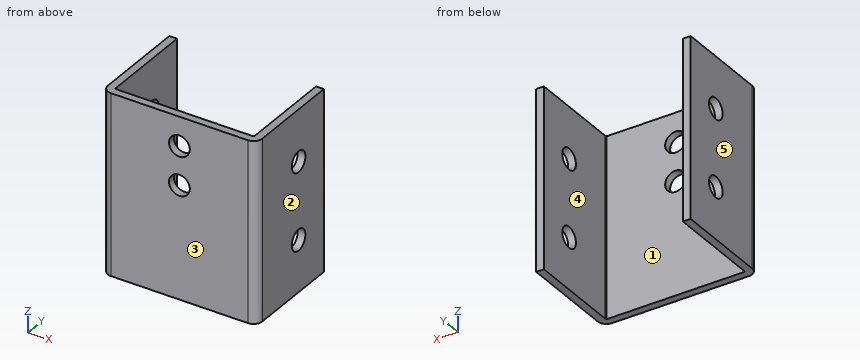
from build123d import *

# Parameters (mm, degrees)
SKETCH1_W                      = 60
SKETCH1_H                      = 70
BASE_FLANGE1_DEPTH             = 3
EDGE_FLANGE1_STRIP_W           = 12.8
EDGE_FLANGE1_STRIP_H           = 3
EDGE_FLANGE1_STRIP_CUT_DEPTH   = 70
EDGE_FLANGE1_STRIP_2_W         = 12.8
EDGE_FLANGE1_STRIP_2_H         = 3
EDGE_FLANGE1_STRIP_CUT_2_DEPTH = 70
EDGE_FLANGE1_DEPTH             = 70
EDGE_FLANGE1_BEND_DEPTH        = 70
CUT_EXTRUDE1_REACH             = 80.702
SKETCH14_R                     = 4.05
SKETCH15_R                     = 4.05
CUT_EXTRUDE2_DEPTH             = 3


# Sheet-metal steps are written as plain solids
with BuildPart() as part:
    # Sketch1 → Base-Flange1 (new body)
    with BuildSketch(Plane(origin=(0, 0, 0), x_dir=(1, 0, 0), z_dir=(0, 1, 0))):
        Rectangle(SKETCH1_W, SKETCH1_H)
    extrude(amount=-BASE_FLANGE1_DEPTH)

    # Edge-Flange1 strip (across the edge) → Edge-Flange1 strip cut (cut)
    with BuildSketch(Plane(origin=(30, 0, 35), x_dir=(-1, 0, 0), z_dir=(0, 0, -1))):
        with Locations((-3, -1.5)):
            Rectangle(EDGE_FLANGE1_STRIP_W, EDGE_FLANGE1_STRIP_H)
    extrude(amount=EDGE_FLANGE1_STRIP_CUT_DEPTH, mode=Mode.SUBTRACT)

    # Edge-Flange1 strip 2 (across the edge) → Edge-Flange1 strip cut 2 (cut)
    with BuildSketch(Plane(origin=(-30, 0, -35), x_dir=(1, 0, 0), z_dir=(0, 0, 1))):
        with Locations((-3, -1.5)):
            Rectangle(EDGE_FLANGE1_STRIP_2_W, EDGE_FLANGE1_STRIP_2_H)
    extrude(amount=EDGE_FLANGE1_STRIP_CUT_2_DEPTH, mode=Mode.SUBTRACT)

    # Edge-Flange1 section (across the edge) → Edge-Flange1 (add)
    with BuildSketch(Plane(origin=(30, 0, 35), x_dir=(-1, 0, 0), z_dir=(0, 0, -1))):
        with BuildLine():
            Line((0, 0.4), (0, 37))
            Line((0, 37), (3, 37))
            Line((3, 37), (3, 0.4))
            ThreePointArc((3, 0.4), (3.117157288, 0.117157288), (3.4, 0))
            Line((3.4, 0), (3.4, -3))
            ThreePointArc((3.4, -3), (0.995836944, -2.004163056), (0, 0.4))
        make_face()
    extrude(amount=EDGE_FLANGE1_DEPTH)

    # Edge-Flange1 section 2 (across the edge) → Edge-Flange1 bend (add)
    with BuildSketch(Plane(origin=(-30, 0, -35), x_dir=(1, 0, 0), z_dir=(0, 0, 1))):
        with BuildLine():
            Line((0, 0.4), (0, 37))
            Line((0, 37), (3, 37))
            Line((3, 37), (3, 0.4))
            ThreePointArc((3, 0.4), (3.117157288, 0.117157288), (3.4, 0))
            Line((3.4, 0), (3.4, -3))
            ThreePointArc((3.4, -3), (0.995836944, -2.004163056), (0, 0.4))
        make_face()
    extrude(amount=EDGE_FLANGE1_BEND_DEPTH)

    # Cut-Extrude1: up to this face of the body (flat: up to its plane)
    cut_extrude1_end = Plane(part.part.faces().sort_by_distance((-30, 18.7, 0))[0])
    # Sketch14 → Cut-Extrude1 (cut, up to the picked face)
    with BuildSketch(Plane(origin=(30, 0, 0), x_dir=(0, 0, -1), z_dir=(1, 0, 0)), mode=Mode.PRIVATE) as cut_extrude1_sk1:
        with Locations(Location((-15, 22, 0), (0, 0, 90))):
            Circle(SKETCH14_R)
    cut_extrude1_tool1 = split(extrude(cut_extrude1_sk1.sketch, amount=-CUT_EXTRUDE1_REACH, mode=Mode.PRIVATE), bisect_by=cut_extrude1_end, keep=Keep.BOTH, mode=Mode.PRIVATE)
    # Sketch14 → Cut-Extrude1 (cut, up to the picked face)
    with BuildSketch(Plane(origin=(30, 0, 0), x_dir=(0, 0, -1), z_dir=(1, 0, 0)), mode=Mode.PRIVATE) as cut_extrude1_sk2:
        with Locations(Location((15, 22, 0), (0, 0, 90))):
            Circle(SKETCH14_R)
    cut_extrude1_tool2 = split(extrude(cut_extrude1_sk2.sketch, amount=-CUT_EXTRUDE1_REACH, mode=Mode.PRIVATE), bisect_by=cut_extrude1_end, keep=Keep.BOTH, mode=Mode.PRIVATE)
    add(cut_extrude1_tool1.solids().sort_by(Axis((30, 22, 15), (-1, 0, 0)))[0], mode=Mode.SUBTRACT)
    add(cut_extrude1_tool2.solids().sort_by(Axis((30, 22, -15), (-1, 0, 0)))[0], mode=Mode.SUBTRACT)

    # Sketch15 → Cut-Extrude2 (cut)
    with BuildSketch(Plane.XZ.offset(3)):
        with Locations(Location((0, 8.75, 0), (0, 0, 270))):
            Circle(SKETCH15_R)
        with Locations(Location((0, 23.75, 0), (0, 0, 270))):
            Circle(SKETCH15_R)
    extrude(amount=-CUT_EXTRUDE2_DEPTH, mode=Mode.SUBTRACT)


solid = part.part
Part model, mm, in its own coordinate system. Face numbers are marked on the shaded views. A direction names the side the tool comes from. Coordinates: 2 decimals unless noted, no trailing zeros. Write each loop counter-clockwise with the first axis right and the second up, starting at its lowest first coordinate (ties: lowest second). Pieces come first, ordered by that corner, then holes. Notation, with made-up numbers: (-18.5, 44) - (27.5, 44) arc R24 cw to (27.5, 83) - close; hole circle Ø7 at (3, -17). An arc over 180 degrees is marked (long way). Put each result on its own line as item: value.
1. Band-saw the part on C-C (x = 0). Write the cut outline in (y, z).
Final values:
outline: (-3, -35) - (0, -35) - (0, 4.7) - (-3, 4.7) - close; (-3, 12.8) - (0, 12.8) - (0, 19.7) - (-3, 19.7) - close; (-3, 27.8) - (0, 27.8) - (0, 35) - (-3, 35) - close
2. Band-saw the part on B-B (y = 34.5). Write the cut outline in (x, z).
Final values:
outline: (-30, -35) - (-27, -35) - (-27, 35) - (-30, 35) - close; (27, -35) - (30, -35) - (30, 35) - (27, 35) - close
3. Probe line 1 along Z through (x, y) = (-29.15, 22); line 2 along X through (y, z) = (11, -28); line 3 along Z through (x, y) = (2, -1). List the from-to ranges inside material, lowest first. Write a range as [from, to].
Final values:
line 1: z = [-35, -19.05], [-10.95, 10.95], [19.05, 35]
line 2: x = [-30, -27], [27, 30]
line 3: z = [-35, 5.23], [12.27, 20.23], [27.27, 35]
4. Two-plate mould, pull along X, no slides. Class the marked faces 1, 2 and 3: +X half, -X half, draft (parallel to the pull), parting line (faces both ways), or undercut.
Final values:
face 1: undercut
face 2: +X half
face 3: draft
5. Band-saw the part on A-A (z = 15). Write the cut outline in (x, y).
Final values:
outline: (-30, 0.4) arc R3.4 ccw to (-26.6, -3) - (26.6, -3) arc R3.4 ccw to (30, 0.4) - (30, 17.95) - (27, 17.95) - (27, 0.4) arc R0.4 cw to (26.6, 0) - (-26.6, 0) arc R0.4 cw to (-27, 0.4) - (-27, 17.95) - (-30, 17.95) - close; (-30, 26.05) - (-27, 26.05) - (-27, 37) - (-30, 37) - close; (27, 26.05) - (30, 26.05) - (30, 37) - (27, 37) - close
6. 3-axis set-ups, long thin cutter, end or side, ignore diameter. For the marked faces 4 and 5: which of +Z, -Z, +X, -X, +Y, -Y reach the whole face in a straight line?
Final values:
face 4: +Z, -Z, +Y
face 5: +Z, -Z, -X, +Y, -Y
7. Flat gauge pins, fed straight in: pin 1 Ø1.5 at (x, z) = (17.5, -15.5) entering from +Y; pin 2 Ø6.5 at (y, z) = (22, 15) entering from -X; pin 3 Ø13 at (y, z) = (22, -15) entering from +X. Where does each tip first touch, or does it go through?
Final values:
pin 1: stops at y = 0
pin 2: passes through
pin 3: stops at x = 30
8. Band-saw the part on D-D (z = -22). Write the cut outline in (x, y), then the cut area to 3 significant figures.
Final values:
outline: (-30, 0.4) arc R3.4 ccw to (-26.6, -3) - (26.6, -3) arc R3.4 ccw to (30, 0.4) - (30, 37) - (27, 37) - (27, 0.4) arc R0.4 cw to (26.6, 0) - (-26.6, 0) arc R0.4 cw to (-27, 0.4) - (-27, 37) - (-30, 37) - close
area: 397 mm²
